from build123d import *

# Parameters (mm, degrees)
SKETCH1_R                = 50
BOSS_EXTRUDE1_DEPTH      = 18
CUT_EXTRUDE1_START       = 5
CUT_EXTRUDE1_DEPTH       = 68.965745388
BOSS_EXTRUDE2_START      = 18
SKETCH1_4_R              = 5.5
BOSS_EXTRUDE2_DEPTH      = 10
BOSS_EXTRUDE3_START      = 28
SKETCH1_5_R              = 5
BOSS_EXTRUDE3_DEPTH      = 15
SKETCH3_R                = 4
CUT_EXTRUDE2_DEPTH       = 18
SKETCH3_3_R              = 4
CUT_EXTRUDE3_DEPTH       = 8
BOSS_EXTRUDE4_REACH      = 159.474
BOSS_EXTRUDE4_END_RADIUS = 50
SKETCH5_W                = 40
SKETCH5_H                = 18
CUT_EXTRUDE4_DEPTH       = 125.088677969
CUT_EXTRUDE5_DEPTH       = 111.625494349
BOSS_EXTRUDE5_START      = 10
SKETCH8_R                = 4
BOSS_EXTRUDE5_DEPTH      = 10


with BuildPart() as part:
    # Sketch1 → Boss-Extrude1 (new body)
    with BuildSketch(Plane(origin=(0, 0, 0), x_dir=(1, 0, 0), z_dir=(0, 1, 0))):
        with Locations(Location((0, 0, 0), (0, 0, 270))):
            Circle(SKETCH1_R)
    extrude(amount=BOSS_EXTRUDE1_DEPTH)

    # Sketch1<3> → Cut-Extrude1 (cut, through all)
    with BuildSketch(Plane(origin=(0, 0, 0), x_dir=(1, 0, 0), z_dir=(0, 1, 0)).offset(CUT_EXTRUDE1_START)):
        with BuildLine():
            ThreePointArc((6.652895641, -39.442857143), (30.545996674, -25.825221919), (40, 0))
            ThreePointArc((40, 0), (30.545996674, 25.825221919), (6.652895641, 39.442857143))
            ThreePointArc((6.652895641, 39.442857143), (7.655820176, 37.321296499), (8, 35))
            ThreePointArc((8, 35), (-2.321296499, 27.344179824), (-6.652895641, 39.442857143))
            ThreePointArc((-6.652895641, 39.442857143), (-28.284271247, 28.284271247), (-39.442857143, 6.652895641))
            ThreePointArc((-39.442857143, 6.652895641), (-31.227922134, 7.054886857), (-27, 0))
            ThreePointArc((-27, 0), (-31.227922134, -7.054886857), (-39.442857143, -6.652895641))
            ThreePointArc((-39.442857143, -6.652895641), (-28.284271247, -28.284271247), (-6.652895641, -39.442857143))
            ThreePointArc((-6.652895641, -39.442857143), (-2.321296499, -27.344179824), (8, -35))
            ThreePointArc((8, -35), (7.655820176, -37.321296499), (6.652895641, -39.442857143))
        make_face()
    extrude(amount=CUT_EXTRUDE1_DEPTH, mode=Mode.SUBTRACT)

    # Sketch1<4> → Boss-Extrude2 (add)
    with BuildSketch(Plane(origin=(0, 0, 0), x_dir=(1, 0, 0), z_dir=(0, 1, 0)).offset(BOSS_EXTRUDE2_START)):
        with Locations(Location((0, 35, 0), (0, 0, 270))):
            Circle(SKETCH1_4_R)
        with Locations(Location((0, -35, 0), (0, 0, 270))):
            Circle(SKETCH1_4_R)
    extrude(amount=BOSS_EXTRUDE2_DEPTH)

    # Sketch1<5> → Boss-Extrude3 (add)
    with BuildSketch(Plane(origin=(0, 0, 0), x_dir=(1, 0, 0), z_dir=(0, 1, 0)).offset(BOSS_EXTRUDE3_START)):
        with Locations(Location((0, 35, 0), (0, 0, 270))):
            Circle(SKETCH1_5_R)
        with Locations(Location((0, -35, 0), (0, 0, 270))):
            Circle(SKETCH1_5_R)
    extrude(amount=BOSS_EXTRUDE3_DEPTH)

    # Sketch3 → Cut-Extrude2 (cut)
    with BuildSketch(Plane.XZ):
        with Locations(Location((0, 35, 0), (0, 0, 270))):
            Circle(SKETCH3_R)
        with Locations(Location((0, -35, 0), (0, 0, 270))):
            Circle(SKETCH3_R)
    extrude(amount=-CUT_EXTRUDE2_DEPTH, mode=Mode.SUBTRACT)

    # Sketch3<3> → Cut-Extrude3 (cut)
    with BuildSketch(Plane.XZ):
        with Locations(Location((-35, 0, 0), (0, 0, 270))):
            Circle(SKETCH3_3_R)
    extrude(amount=-CUT_EXTRUDE3_DEPTH, mode=Mode.SUBTRACT)

    # Boss-Extrude4: up to this cylinder (the profile starts outside it)
    boss_extrude4_end = Plane(origin=(0, 9, 0), z_dir=(0, -1, 0)) * Cylinder(BOSS_EXTRUDE4_END_RADIUS, 419.948, mode=Mode.PRIVATE)
    # Sketch5 → Boss-Extrude4 (add, up to the surface)
    with BuildSketch(Plane(origin=(93, 0, 0), x_dir=(0, 0, -1), z_dir=(1, 0, 0)), mode=Mode.PRIVATE) as boss_extrude4_sk1:
        with Locations((0, 9)):
            Rectangle(SKETCH5_W, SKETCH5_H)
    boss_extrude4_tool1 = extrude(boss_extrude4_sk1.sketch, amount=-BOSS_EXTRUDE4_REACH, mode=Mode.PRIVATE) - boss_extrude4_end
    add(boss_extrude4_tool1.solids().sort_by_distance((93, 9, 0))[0])

    # Sketch6 → Cut-Extrude4 (cut, through all)
    with BuildSketch(Plane.XY.offset(20)):
        Polygon((93, 10), (63, 10), (45.82575695, 18), (93, 18), align=None)
    extrude(amount=-CUT_EXTRUDE4_DEPTH, mode=Mode.SUBTRACT)

    # Sketch7 → Cut-Extrude5 (cut, through all)
    with BuildSketch(Plane(origin=(0, 10, 0), x_dir=(1, 0, 0), z_dir=(0, 1, 0))):
        Polygon((63, 20), (93, 10), (93, 20), align=None)
        Polygon((93, -10), (93, -20), (63, -20), align=None)
    extrude(amount=-CUT_EXTRUDE5_DEPTH, mode=Mode.SUBTRACT)

    # Sketch8 → Boss-Extrude5 (add)
    with BuildSketch(Plane.XY.offset(BOSS_EXTRUDE5_START)):
        with BuildLine():
            Line((12.173938425, 0), (24.875644347, -22))
            ThreePointArc((24.875644347, -22), (40.623466631, -28.522961568), (51, -15))
            Line((51, -15), (51, 0))
            Line((51, 0), (12.173938425, 0))
        make_face()
        with Locations((37, -15)):
            Circle(SKETCH8_R, mode=Mode.SUBTRACT)
    boss_extrude5 = extrude(amount=BOSS_EXTRUDE5_DEPTH)

    # Mirror1: Boss-Extrude5 across plane
    add(boss_extrude5.mirror(Plane.XY))


solid = part.part
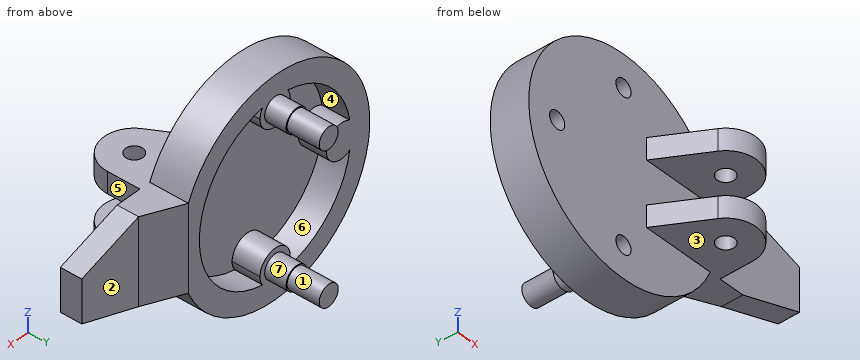
CAD build for the part. Positions are in the model's coordinates, mm. Face numbers are marked on the shaded views. A direction names the side the tool comes from. Round coordinates to 2 decimals unless told otherwise and drop trailing zeros. Write each loop counter-clockwise with the first axis right and the second up, starting at its lowest first coordinate (ties: lowest second). Pieces come first, ordered by that corner, then holes. Notation, with made-up numbers: (77, 63.5) -> (104, 63.5) arc R27 ccw to (104, 96.5) -> close; hole circle Ø7 at (-14, -30). An arc over 180 degrees is marked (long way). Answer as a JSON object with one key per item and string values.
(1) Which spindle directions (+Z, -Z, +X, -X, +Y, -Y) get a long thin tool onto all of the face, cutting with end or side? Do the marked faces 1, 2 and 3. Say none if no direction does.
Reported:
{"face 1": "+Y", "face 2": "+Z, -Z, +X, +Y", "face 3": "-Z, +X, -Y"}
(2) Probe probe 1 along X at (y, z) = (6, 0); probe 2 along Y at (x, z) = (37, -12); probe 3 along X at (y, z) = (7, -35). List the from-to ranges inside material, lowest first. Write a range as [from, to].
Reported:
{"probe 1": "x = [-50, -39], [-31, -27], [40, 93]", "probe 2": "y = [-29, -19], [-11, 5]", "probe 3": "x = [-35.71, -19.36], [-8, -4], [4, 8], [19.36, 35.71]"}
(3) Band-saw the part on B-B, the plane y = 25. List the corners of the cut face in (x, z).
Reported:
{"outline": "circle Ø11 at (0, -35); circle Ø11 at (0, 35)"}
(4) Two-plate mould, pull along X, no slides. Class the marked faces 4, 5, 6 and 7: +X half, -X half, draft (parallel to the pull), parting line (faces both ways), or undercut.
Reported:
{"face 4": "undercut", "face 5": "+X half", "face 6": "undercut", "face 7": "parting line"}
(5) Pin check, flat tips, straight feed: P1, Ø4, axis at y = 27.5, z = -34.5, coming from the +X side; P2, Ø14.5, axis at x = 39.5, y = -13, coming from the +Z side; P3, Ø12, axis at x = -27.5, y = 22.5, coming from the -Z side; P4, Ø5, axis at x = 37, y = -15, coming from the -Z side. Stop position of each tip, or through.
Reported:
{"P1": "stops at x = 5.5", "P2": "stops at z = 20", "P3": "stops at z = -44.12", "P4": "passes through"}
(6) Band-saw the part on C-C, the plane x = 37. List the corners of the cut face in (y, z).
Reported:
{"outline": "(-29, -20) -> (-19, -20) -> (-19, -10) -> (-29, -10) -> close; (-29, 10) -> (-19, 10) -> (-19, 20) -> (-29, 20) -> close; (-11, -20) -> (0, -20) -> (0, -33.63) -> (18, -33.63) -> (18, -15.2) -> (5, -15.2) -> (5, 15.2) -> (18, 15.2) -> (18, 33.63) -> (0, 33.63) -> (0, 20) -> (-11, 20) -> (-11, 10) -> (0, 10) -> (0, -10) -> (-11, -10) -> close"}
(7) Band-saw the part on D-D, the plane z = 37. List the corners of the cut face in (x, y), then the cut area to 3 significant figures.
Reported:
{"outline": "(-33.63, 0) -> (-3.46, 0) -> (-3.46, 18) -> (3.46, 18) -> (3.46, 0) -> (33.63, 0) -> (33.63, 18) -> (15.2, 18) -> (15.2, 5) -> (7.75, 5) -> (7.75, 18) -> (5.12, 18) -> (5.12, 28) -> (4.58, 28) -> (4.58, 43) -> (-4.58, 43) -> (-4.58, 28) -> (-5.12, 28) -> (-5.12, 18) -> (-7.75, 18) -> (-7.75, 5) -> (-15.2, 5) -> (-15.2, 18) -> (-33.63, 18) -> close", "area": "1,130 mm^2"}
